Input: part model. Units: mm. Frame: model coordinates. Face numbers are marked on the shaded views. Round coordinates to 2 decimals unless told otherwise and drop trailing zeros. Write each loop counter-clockwise with the first axis right and the second up, starting at its lowest first coordinate (ties: lowest second). Pieces come first, ordered by that corner, then holes. Notation, with made-up numbers: (-9.75, 16) -> (7.25, 16) arc R30 ccw to (7.25, 50) -> close; hole circle Ø7 at (87.5, -1). An arc over 180 degrees is marked (long way). Use CSV: the item, a comma, the result in double quotes.
```python
from build123d import *

# Parameters (mm, degrees)
SM_BASE_FLANGE_1_DEPTH   = 3
OTHER_START              = 10
OTHER_1_DEPTH            = 10
OTHER_START_2            = -20
OTHER_2_DEPTH            = 10
HOLE_WIZARD_1_AT_2_COUNT = 2
HOLE_WIZARD_1_AT_2_PITCH = 24
SKETCH_12_W              = 100
SKETCH_12_H              = 20
EXTRUDE_1_DEPTH          = 10
FILLET_1_R               = 5
SKETCH_13_R              = 2.5
EXTRUDE_2_DEPTH          = 3
FILLET_2_R               = 2


# Read off the part's stored shape, not the designer's step: 褶边1, 褶边2
# Sheet-metal steps are written as plain solids
with BuildPart() as part:
    # Sketch 1 → 基体-法兰1 (new body)
    with BuildSketch(Plane(origin=(0, 0, 0), x_dir=(1, 0, 0), z_dir=(0, 1, 0))):
        with BuildLine():
            Line((-25, -12.5), (25, -12.5))
            Line((25, -12.5), (25, 7.5))
            ThreePointArc((25, 7.5), (23.535533906, 11.035533906), (20, 12.5))
            Line((20, 12.5), (-20, 12.5))
            ThreePointArc((-20, 12.5), (-23.535533906, 11.035533906), (-25, 7.5))
            Line((-25, 7.5), (-25, -12.5))
        make_face()
    extrude(amount=-SM_BASE_FLANGE_1_DEPTH)

    # Other 1 outline → Other 1 (add)
    with BuildSketch(Plane.YZ.offset(OTHER_START)):
        with BuildLine():
            Line((2, 10.5), (2, 7.5))
            ThreePointArc((2, 7.5), (5.535533906, 16.035533906), (-3, 12.5))
            Line((-3, 12.5), (0, 12.5))
            ThreePointArc((0, 12.5), (3.414213562, 13.914213562), (2, 10.5))
        make_face()
    extrude(amount=OTHER_1_DEPTH)

    # Other 2 outline → Other 2 (add)
    with BuildSketch(Plane.YZ.offset(OTHER_START_2)):
        with BuildLine():
            Line((2, 10.5), (2, 7.5))
            ThreePointArc((2, 7.5), (5.535533906, 16.035533906), (-3, 12.5))
            Line((-3, 12.5), (0, 12.5))
            ThreePointArc((0, 12.5), (3.414213562, 13.914213562), (2, 10.5))
        make_face()
    extrude(amount=OTHER_2_DEPTH)

    # 草图11 → 打孔尺寸(%根据十字)槽半沉头木螺钉的类型1 (revolve, cut)
    with BuildSketch(Plane(origin=(-12, 0, 0), x_dir=(0, 0, 1), z_dir=(1, 0, 0))):
        Polygon((0, 0), (0, 3), (2.25, 3), (2.25, 2.05), (4.3, 0), align=None)
    hole_wizard_1 = revolve(axis=Axis((-12, 6.35, 0), (0, -1, 0)), mode=Mode.SUBTRACT)

    # 打孔尺寸(%根据十字)槽半沉头木螺钉的类型1 at 2: 打孔尺寸(%根据十字)槽半沉头木螺钉的类型1 ×2
    with Locations(*[(i * HOLE_WIZARD_1_AT_2_PITCH, 0, 0) for i in range(1, HOLE_WIZARD_1_AT_2_COUNT)]):
        add(hole_wizard_1, mode=Mode.SUBTRACT)

    # 草图12 → 凸台-拉伸1 (add)
    with BuildSketch(Plane(origin=(0, -3, 0), x_dir=(1, 0, 0), z_dir=(0, 1, 0))):
        Rectangle(SKETCH_12_W, SKETCH_12_H)
    extrude(amount=-EXTRUDE_1_DEPTH)

    # 圆角1
    fillet_1_edges = [part.edges().sort_by_distance(p)[0] for p in [
        (50, -13, 0),
        (-50, -13, 0),
        (0, -13, -10),
    ]]
    fillet(fillet_1_edges, radius=FILLET_1_R)

    # 草图13 → 凸台-拉伸2 (add)
    with BuildSketch(Plane.XY.offset(10)):
        with Locations((-25, -7.95945711)):
            Circle(SKETCH_13_R)
        with Locations((0, -7.95945711)):
            Circle(SKETCH_13_R)
        with Locations((25, -7.95945711)):
            Circle(SKETCH_13_R)
    extrude(amount=EXTRUDE_2_DEPTH)

    # 圆角2
    fillet_2_edges = [part.edges().sort_by_distance(p)[0] for p in [
        (22.5, -7.95945711, 13),
        (-27.5, -7.95945711, 13),
    ]]
    fillet(fillet_2_edges, radius=FILLET_2_R)


solid = part.part
```
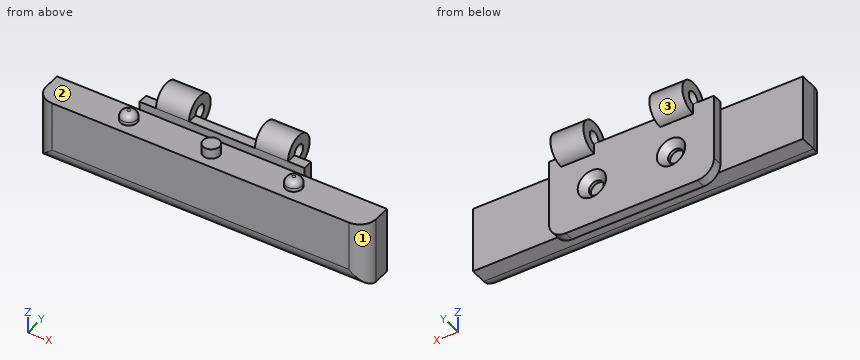
Item 1: Pull-direction query (X, two-part tool) for the marked faces 1, 2 and 3; classes: +X half, -X half, draft (parallel to the pull), parting line (faces both ways), or undercut.
Worked answers:
face 1,"+X half"
face 2,"undercut"
face 3,"draft"
Item 2: Line query: line 1 (X direction, y = -2.8, z = 0); line 2 (X direction, y = -0.5, z = 14); line 3 (Y direction, x = -13.5, z = 12.5). Output: solid intervals per line, ascending.
Worked answers:
line 1,"x = -25 to -14.25, -9.75 to 9.75, 14.25 to 25"
line 2,"x = -20 to -10, 10 to 20"
line 3,"y = -3 to 0, 4 to 7"
Item 3: Section query C-C on z = 0. Return the cut outline in (x, y), plus the area to 3 significant figures.
Worked answers:
outline,"(-50, -8) arc R5 ccw to (-45, -13) -> (45, -13) arc R5 ccw to (50, -8) -> (50, -3) -> (25, -3) -> (25, 0) -> (16.3, 0) -> (14.25, -2.05) -> (14.25, -3) -> (9.75, -3) -> (9.75, -2.05) -> (7.7, 0) -> (-7.7, 0) -> (-9.75, -2.05) -> (-9.75, -3) -> (-14.25, -3) -> (-14.25, -2.05) -> (-16.3, 0) -> (-25, 0) -> (-25, -3) -> (-50, -3) -> close"
area,"1,100 mm²"
Item 4: Section query D-D on x = 40. Return the cut outline in (y, z), plus the area to 3 significant figures.
Worked answers:
outline,"(-13, -5) arc R5 ccw to (-8, -10) -> (-3, -10) -> (-3, 10) -> (-13, 10) -> close"
area,"195 mm²"
Item 5: Section query A-A on z = 6. Return the cut outline in (x, y), plus the area to 3 significant figures.
Worked answers:
outline,"(-50, -8) arc R5 ccw to (-45, -13) -> (45, -13) arc R5 ccw to (50, -8) -> (50, -3) -> (25, -3) -> (25, 0) -> (-25, 0) -> (-25, -3) -> (-50, -3) -> close"
area,"1,140 mm²"
Item 6: First-contact query: pin 1 Ø6 at (x, z) = (15, -8.5) entering from -Y; pin 2 Ø11 at (y, z) = (2, 13.5) entering from -X; pin 3 Ø1.5 at (x, y) = (-23, -2) entering from +Z. Flat tips, straight axial feed; report the tip coordinate or a pass-through.
Worked answers:
pin 1,"stops at y = -12.97"
pin 2,"stops at x = -25"
pin 3,"stops at z = 12.5"
Item 7: Section query B-B on x = 0. Return the cut outline in (y, z), plus the area to 3 significant figures.
Worked answers:
outline,"(-13, -5) arc R5 ccw to (-8, -10) -> (-3, -10) -> (-3, -12.5) -> (0, -12.5) -> (0, 12.5) -> (-3, 12.5) -> (-3, 10) -> (-5.46, 10) -> (-5.46, 13) -> (-10.46, 13) -> (-10.46, 10) -> (-13, 10) -> close"
area,"285 mm²"
